Verification items for the finished model (mm, model axes). A direction names the side the tool comes from. Give positions to 0.01 mm unless a question says otherwise; leave off trailing zeros. Loops run counter-clockwise (first coordinate to the right, second up) from the corner with the lowest first, then second, coordinate; pieces in that order, holes last. Notation, with made-up numbers: M 12.5,15 L 59.5,15 A28 cw 59.5,36 Z; hole C -31.5,22 d11. An arc over 180 degrees is marked long. Use a Markdown table: item, result.
from build123d import *

# Parameters (mm, degrees)
SKETCH_W        = 40
SKETCH_H        = 85
PAD_DEPTH       = 50
POCKET_DEPTH    = 50
POCKET001_DEPTH = 25
SKETCH004_W     = 16
SKETCH004_H     = 26
POCKET002_DEPTH = 18
SKETCH005_R     = 2
POCKET003_DEPTH = 4
POCKET005_DEPTH = 18
SKETCH008_W     = 34
SKETCH008_H     = 62
POCKET006_DEPTH = 32
SKETCH009_R     = 5.95
SKETCH009_R_2   = 4.5
POCKET007_DEPTH = 18.001
SKETCH010_R     = 10.85
POCKET008_DEPTH = 8
POCKET009_DEPTH = 40.001
SKETCH012_R     = 2
POCKET010_DEPTH = 5


with BuildPart() as part:
    # Sketch → Pad (new body)
    with BuildSketch(Plane.YZ):
        Rectangle(SKETCH_W, SKETCH_H)
    extrude(amount=PAD_DEPTH)

    # Sketch001 (on Face6 of Pad) → Pocket (cut)
    with BuildSketch(Plane.YZ.offset(50)):
        Polygon((0, -22.5), (0, -42.5), (20, -42.5), (20, -22.5), (12.48396, -22.5), (12.48396, -24.5), (15.18396, -24.5), (12, -27.68), (8, -27.68), (4.81604, -24.5), (7.51604, -24.5), (7.51604, -22.5), align=None)
    extrude(amount=-POCKET_DEPTH, mode=Mode.SUBTRACT)

    # Sketch003 (on Face2 of Pocket) → Pocket001 (cut)
    with BuildSketch(Plane(origin=(0, -20, 0), x_dir=(0, 0, -1), z_dir=(0, -1, 0))):
        Polygon((42.5, 50), (22.5, 50), (22.5, 42.48), (24.5, 42.48), (24.5, 45.18), (27.68, 42), (27.68, 38), (24.5, 34.82), (24.5, 37.52), (22.5, 37.52), (22.5, 30), (42.5, 30), align=None)
    extrude(amount=-POCKET001_DEPTH, mode=Mode.SUBTRACT)

    # Sketch004 (on Face2 of Pocket001) → Pocket002 (cut)
    with BuildSketch(Plane(origin=(0, -20, 0), x_dir=(0, 0, -1), z_dir=(0, -1, 0))):
        with Locations((32.5, 13)):
            Rectangle(SKETCH004_W, SKETCH004_H)
    extrude(amount=-POCKET002_DEPTH, mode=Mode.SUBTRACT)

    # Sketch005 (on Face30 of Pocket002) → Pocket003 (cut)
    with BuildSketch(Plane(origin=(0, -2, 0), x_dir=(0, 0, -1), z_dir=(0, -1, 0))):
        with Locations((32.5, 13)):
            Circle(SKETCH005_R)
    extrude(amount=-POCKET003_DEPTH, mode=Mode.SUBTRACT)

    # Sketch007 → Pocket005 (cut)
    with BuildSketch(Plane.YX.offset(42.5)):
        Polygon((-25.002718, 26), (-25, 0), (0, 0), align=None)
    extrude(amount=-POCKET005_DEPTH, mode=Mode.SUBTRACT)

    # Sketch008 (on Face5 of Pocket005) → Pocket006 (cut)
    with BuildSketch(Plane.YZ.offset(50)):
        with Locations((0, 11.5)):
            Rectangle(SKETCH008_W, SKETCH008_H)
    extrude(amount=-POCKET006_DEPTH, mode=Mode.SUBTRACT)

    # Sketch009 (on Face6 of Pocket006) → Pocket007 (cut, through all)
    with BuildSketch(Plane.YZ.offset(18)):
        with Locations((0, 23.5)):
            Circle(SKETCH009_R)
        with Locations((0.095747, 1.5)):
            Circle(SKETCH009_R_2)
    extrude(amount=-POCKET007_DEPTH, mode=Mode.SUBTRACT)

    # Sketch010 (on Face2 of Pocket007) → Pocket008 (cut)
    with BuildSketch(Plane(origin=(0, 0, 0), x_dir=(0, 1, 0), z_dir=(-1, 0, 0))):
        with Locations((0.095747, -1.5)):
            Circle(SKETCH010_R)
    extrude(amount=-POCKET008_DEPTH, mode=Mode.SUBTRACT)

    # Sketch011 (on Face3 of Pocket008) → Pocket009 (cut, through all)
    with BuildSketch(Plane.ZX.offset(20)):
        Polygon((-17.5, 50), (42.5, 25), (42.5, 50), align=None)
    extrude(amount=-POCKET009_DEPTH, mode=Mode.SUBTRACT)

    # Sketch012 (on Face29 of Pocket009) → Pocket010 (cut)
    with BuildSketch(Plane(origin=(26, 0, 0), x_dir=(0, 1, 0), z_dir=(-1, 0, 0))):
        with Locations((-11, 32.5)):
            Circle(SKETCH012_R)
    extrude(amount=-POCKET010_DEPTH, mode=Mode.SUBTRACT)


solid = part.part
(1) Cross-section at D-D on z = 23.5. Record the cut outline in (x, y), then the cut area to 3 significant figures.
Results below:
| item | result |
|---|---|
| outline | M 0,-20 L 32.92,-20 L 32.92,-17 L 18,-17 L 18,-5.95 L 0,-5.95 Z; M 0,5.95 L 18,5.95 L 18,17 L 32.92,17 L 32.92,20 L 0,20 Z |
| area | 595 mm^2 |
(2) Draft check along Z on faces 1 (the flat face through (25.35, 6.43, -26.11)), 2 (the flat face through (19, 20, 2)), 3 (the flat face through (26, -13, -34)). Enter one of: +Z half, -Z half, draft (parallel to the pull), parting line (faces both ways), or undercut.
Results below:
| item | result |
|---|---|
| face 1 | -Z half |
| face 2 | draft |
| face 3 | undercut |
(3) Cross-section at C-C on y = 13.5. Record the cut outline in (x, z).
Results below:
| item | result |
|---|---|
| outline | M 0,-26.18 L 50,-26.18 L 50,-24.5 L 0,-24.5 Z; M 0,-22.5 L 50,-22.5 L 50,-19.5 L 18,-19.5 L 18,42.5 L 0,42.5 Z |
(4) Gauge pin test, flat ends, axial feed: P1, Ø6.5, axis at x = 13, z = -32.5, coming from the -Y side; P2, Ø12, axis at y = 11.5, z = 24, coming from the -X side; P3, Ø2, axis at x = 23.5, y = 9.5, coming from the -Z side; P4, Ø1.6, axis at x = 39.5, z = -26, coming from the +Y side. Record the tip position at first contact, or that the pin passes through.
Results below:
| item | result |
|---|---|
| P1 | y = -2 |
| P2 | x = 0 |
| P3 | z = -27.68 |
| P4 | y = 14.48 |
(5) Cross-section at B-B on x = 40.5. Record the cut outline in (y, z), then the cut area to 3 significant figures.
Results below:
| item | result |
|---|---|
| outline | M -20,-27.68 L 0,-27.68 L 0,-22.5 L 7.52,-22.5 L 7.52,-24.5 L 4.82,-24.5 L 8,-27.68 L 12,-27.68 L 15.18,-24.5 L 12.48,-24.5 L 12.48,-22.5 L 20,-22.5 L 20,5.3 L 17,5.3 L 17,-19.5 L -17,-19.5 L -17,5.3 L -20,5.3 Z |
| area | 405 mm^2 |
(6) Set-up check for faces 4 (the flat face through (8, -0.1, 6.2)), 5 (the flat face through (31, -3, -22.5)), 6 (the flat face through (34, 0, -19.5)), 7 (the flat face through (40, 0, -25)), 8 (the flat face through (25, 14, -24.5)): record each of +Z, -Z, +X, -X, +Y, -Y from which the full face is reachable in a straight line by a thin tool's end or side.
Results below:
| item | result |
|---|---|
| face 4 | -X |
| face 5 | none |
| face 6 | +Z, +X |
| face 7 | -Z, +X, -X |
| face 8 | +X, -X, +Y |
(7) Material ranges on line 1 (Y direction, x = 4, z = 1); line 2 (Z direction, x = 3, y = -0.5); line 3 (Y direction, x = 32.5, z = 20), recorded low to high.
Results below:
| item | result |
|---|---|
| line 1 | -20 to -10.74, 10.93 to 20 |
| line 2 | -42.5 to -9.33, 12.33 to 17.57, 29.43 to 42.5 |
| line 3 | -20 to -17, 17 to 20 |
(8) Cross-section at A-A on z = -32.5. Record the cut outline in (x, y), then the cut area to 3 significant figures.
Results below:
| item | result |
|---|---|
| outline | M 0,0 L 2.08,-2 L 11,-2 L 11,0 Z; M 15,-2 L 26,-2 L 26,-9 L 30,-9 L 30,0 L 15,0 Z; M 26,-20 L 30,-20 L 30,-13 L 26,-13 Z |
| area | 106 mm^2 |
